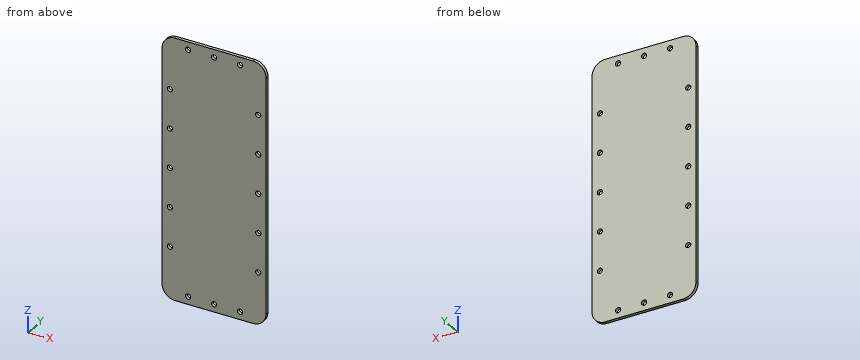
```python
from build123d import *

# Parameters (mm, degrees)
SKETCH1_W           = 101.6
SKETCH1_H           = 254
BOSS_EXTRUDE1_DEPTH = 3.175
SKETCH2_R           = 2.54
CUT_EXTRUDE1_DEPTH  = 223.663234681
FILLET1_R           = 12.7


with BuildPart() as part:
    # Sketch1 → Boss-Extrude1 (new body)
    with BuildSketch(Plane(origin=(0, 0, 0), x_dir=(1, 0, 0), z_dir=(0, 1, 0))):
        with Locations((20.100372359, -84.049692378)):
            Rectangle(SKETCH1_W, SKETCH1_H)
    extrude(amount=BOSS_EXTRUDE1_DEPTH)

    # Sketch2 → Cut-Extrude1 (cut, through all)
    with BuildSketch(Plane(origin=(0, 3.175, 0), x_dir=(1, 0, 0), z_dir=(0, 1, 0))):
        with Locations(Location((-5.299627641, 35.330307622, 0), (0, 0, 270))):
            Circle(SKETCH2_R)
        with Locations(Location((20.100372359, 35.330307622, 0), (0, 0, 270))):
            Circle(SKETCH2_R)
        with Locations(Location((45.500372359, 35.330307622, 0), (0, 0, 270))):
            Circle(SKETCH2_R)
        with Locations(Location((-23.079627641, -84.049692378, 0), (0, 0, 270))):
            Circle(SKETCH2_R)
        with Locations(Location((-23.079627641, -45.949692378, 0), (0, 0, 270))):
            Circle(SKETCH2_R)
        with Locations(Location((-23.079627641, -7.849692378, 0), (0, 0, 270))):
            Circle(SKETCH2_R)
        with Locations(Location((63.280372359, -7.849692378, 0), (0, 0, 90))):
            Circle(SKETCH2_R)
        with Locations(Location((63.280372359, -45.949692378, 0), (0, 0, 90))):
            Circle(SKETCH2_R)
        with Locations(Location((63.280372359, -84.049692378, 0), (0, 0, 90))):
            Circle(SKETCH2_R)
        with Locations(Location((63.280372359, -122.149692378, 0), (0, 0, 270))):
            Circle(SKETCH2_R)
        with Locations(Location((63.280372359, -160.249692378, 0), (0, 0, 270))):
            Circle(SKETCH2_R)
        with Locations(Location((-23.079627641, -160.249692378, 0), (0, 0, 90))):
            Circle(SKETCH2_R)
        with Locations(Location((-23.079627641, -122.149692378, 0), (0, 0, 90))):
            Circle(SKETCH2_R)
        with Locations(Location((45.500372359, -203.429692378, 0), (0, 0, 90))):
            Circle(SKETCH2_R)
        with Locations(Location((20.100372359, -203.429692378, 0), (0, 0, 90))):
            Circle(SKETCH2_R)
        with Locations(Location((-5.299627641, -203.429692378, 0), (0, 0, 90))):
            Circle(SKETCH2_R)
    extrude(amount=-CUT_EXTRUDE1_DEPTH, mode=Mode.SUBTRACT)

    # Fillet1
    fillet1_edges = [part.edges().sort_by_distance(p)[0] for p in [
        (-30.699627641, 1.5875, -42.950307622),
        (70.900372359, 1.5875, -42.950307622),
        (70.900372359, 1.5875, 211.049692378),
        (-30.699627641, 1.5875, 211.049692378),
    ]]
    fillet(fillet1_edges, radius=FILLET1_R)


solid = part.part
```
Source: CAD feature listing. Evaluate the final solid. Frame: model axes, mm. Give positions to 0.01 mm unless a question says otherwise; leave off trailing zeros.
(1) Material intervals for line 1 along X through (y, z) = (2.7, 8); line 2 along Z through (x, y) = (-4, 2.25); line 3 along Z through (x, y) = (64, 0.9), sorted ascending.
(2) Contact query for a flat-ended pin moving along its axis: P1, Ø4, axis at x = 45.5, z = 203.43, coming from the +Y side. Output: stop coordinate, or through.
(3) Section query A-A (y = 0.5). State how many separate pieces and enclosed holes the cut face has, plus the area to 3 significant figures.
Outcome:
1. line 1: x = -30.7 to -25.62, -20.54 to 60.74, 65.82 to 70.9
1. line 2: z = -42.95 to -37.51, -33.15 to 201.25, 205.61 to 211.05
1. line 3: z = -41.55 to 5.41, 10.29 to 43.51, 48.39 to 81.61, 86.49 to 119.71, 124.59 to 157.81, 162.69 to 209.65
2. P1: passes through
3. separate pieces: 1
3. enclosed holes: 16
3. area: 25,300 mm2
